Geometry: final body of the model. Coordinates: model frame, mm. Coordinates: 2 decimals unless noted, no trailing zeros. Order: outer loops, then holes, each group sorted by start corner. A loop starts at its lowest first (then second) coordinate and runs counter-clockwise, first axis right, second up. Notation, with made-up numbers: M 3.25,86 L 44.25,86 A24 ccw 44.25,112 Z; hole C 38,-20 d6. An arc over 180 degrees is marked long. One line per question, with ' | ' between items.
from build123d import *

# Parameters (mm, degrees)
SALIENTE_EXTRUIR1_DEPTH = 3
CROQUIS3_R              = 8
CORTAR_EXTRUIR2_DEPTH   = 3
CROQUIS5_W              = 9.084
CROQUIS5_H              = 3
SALIENTE_EXTRUIR2_DEPTH = 3


with BuildPart() as part:
    # Croquis1 → Saliente-Extruir1 (new body)
    with BuildSketch(Plane.XY):
        with BuildLine():
            Line((-22.71, -10.17), (22.71, -10.17))
            Line((22.71, -10.17), (22.71, 7.83))
            ThreePointArc((22.71, 7.83), (19.781067812, 14.901067812), (12.71, 17.83))
            Line((12.71, 17.83), (-12.71, 17.83))
            ThreePointArc((-12.71, 17.83), (-19.781067812, 14.901067812), (-22.71, 7.83))
            Line((-22.71, 7.83), (-22.71, -10.17))
        make_face()
    extrude(amount=SALIENTE_EXTRUIR1_DEPTH)

    # Croquis3 → Cortar-Extruir2 (cut)
    with BuildSketch(Plane.XY.offset(3)):
        with Locations((-13, 7.65)):
            Circle(CROQUIS3_R)
        with Locations((13, 7.65)):
            Circle(CROQUIS3_R)
    extrude(amount=-CORTAR_EXTRUIR2_DEPTH, mode=Mode.SUBTRACT)

    # Croquis5 → Saliente-Extruir2 (add)
    with BuildSketch(Plane.XZ.offset(10.17)):
        with Locations((-18.168, 1.5)):
            Rectangle(CROQUIS5_W, CROQUIS5_H)
        with Locations((0, 1.5)):
            Rectangle(CROQUIS5_W, CROQUIS5_H)
        with Locations((18.168, 1.5)):
            Rectangle(CROQUIS5_W, CROQUIS5_H)
    extrude(amount=SALIENTE_EXTRUIR2_DEPTH)


solid = part.part
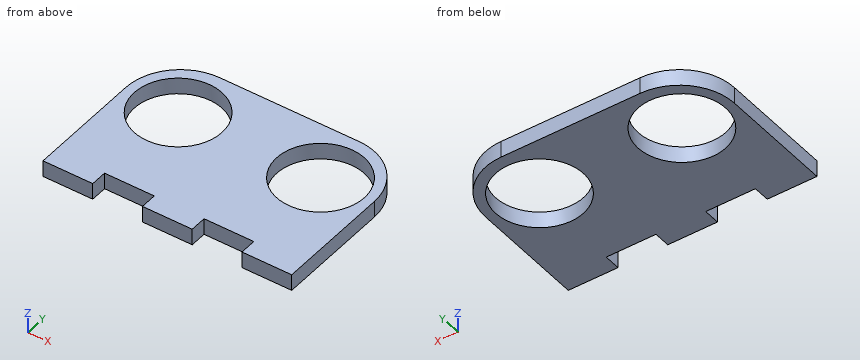
1. Section A-A, the plane y = 1.5. Output: boundary loops of the cut face in (x, z), and give its area (3 significant figures).
Response values:
outline: M -22.71,0 L -18.12,0 L -18.12,3 L -22.71,3 Z; M -7.88,0 L 7.88,0 L 7.88,3 L -7.88,3 Z; M 18.12,0 L 22.71,0 L 22.71,3 L 18.12,3 Z | area: 74.9 mm^2
2. Pin query (flat end, axial travel): P1, Ø1, axis at y = 11, z = 2, coming from the +X side; P2, Ø1, axis at x = -15, z = 1.5, coming from the +Y side. Return the tip coordinate at first contact, or that it passes through.
Response values:
P1: stops at x = 22.35 | P2: stops at y = 17.67
3. Section B-B, the plane x = 9. Output: boundary loops of the cut face in (y, z), and give its area (3 significant figures).
Response values:
outline: M -10.17,0 L 0.72,0 L 0.72,3 L -10.17,3 Z; M 14.58,0 L 17.83,0 L 17.83,3 L 14.58,3 Z | area: 42.4 mm^2
4. Section C-C, the plane z = 0.55. Output: boundary loops of the cut face in (x, y).
Response values:
outline: M -22.71,-13.17 L -13.63,-13.17 L -13.63,-10.17 L -4.54,-10.17 L -4.54,-13.17 L 4.54,-13.17 L 4.54,-10.17 L 13.63,-10.17 L 13.63,-13.17 L 22.71,-13.17 L 22.71,7.83 A10 ccw 12.71,17.83 L -12.71,17.83 A10 ccw -22.71,7.83 Z; hole C -13,7.65 d16; hole C 13,7.65 d16
5. Material intervals for line 1 (Y direction, x = 13, z = 1.7); line 2 (X direction, y = 8, z = 2.85); line 3 (X direction, y = 13, z = 1.6), sorted ascending. Write a range as [from, to].
Response values:
line 1: y = [-10.17, -0.35], [15.65, 17.83] | line 2: x = [-22.71, -20.99], [-5.01, 5.01], [20.99, 22.71] | line 3: x = [-21.27, -18.95], [-7.05, 7.05], [18.95, 21.27]
6. Section D-D, the plane y = 15. Output: boundary loops of the cut face in (x, z), and give its area (3 significant figures).
Response values:
outline: M -19.68,0 L -16.16,0 L -16.16,3 L -19.68,3 Z; M -9.84,0 L 9.84,0 L 9.84,3 L -9.84,3 Z; M 16.16,0 L 19.68,0 L 19.68,3 L 16.16,3 Z | area: 80.2 mm^2
